```python
from build123d import *

# Parameters (mm, degrees)
F0_W     = 76.2
F0_H     = 254
F0_R     = 6.35
F1_DEPTH = 25.4
F2_R     = 38.09999


# Not quite as in the source:
# - a fillet or chamfer is up to 0.001 mm smaller than in the source, because OpenCascade refuses the exact size


with BuildPart() as f1:
    # F0 (on Front) → F1 (new body)
    with BuildSketch(Plane.XZ):
        with Locations((-38.1, 127)):
            Rectangle(F0_W, F0_H)
        with Locations((-38.1, 228.6)):
            Circle(F0_R, mode=Mode.SUBTRACT)
    extrude(amount=F1_DEPTH)

    # F2 (radius 38.1 in the source; OpenCascade refuses exactly that, so slightly less here)
    f2_edges = [f1.edges().sort_by_distance(p)[0] for p in [
        (-76.2, -12.7, 254),
        (0, -12.7, 254),
    ]]
    fillet(f2_edges, radius=F2_R)


solid = f1.part
```
Could you check a few things on this model? Use its own coordinates, in mm. Give positions to 0.01 mm unless a question says otherwise; leave off trailing zeros. Write each loop counter-clockwise with the first axis right and the second up, starting at its lowest first coordinate (ties: lowest second). Pieces come first, ordered by that corner, then holes. Notation, with made-up numbers: (-25, 73.25) -> (22, 73.25) arc R23 ccw to (22, 86.25) -> close; hole circle Ø7 at (9, 73.25). An arc over 180 degrees is marked (long way). Write each question's results on one line, items separated by ' | '.
1. I need wall thicknesses on L1, parallel to X at y = -18, z = 224.5; L2, parallel to Z at x = -58, y = -18; L3, parallel to Z at x = -36.5, y = -15.25. Which ranges of each line are inside material? Lowest first, please.
Check sheet entries:
L1: x = -75.22 to -42.95, -33.25 to -0.98 | L2: z = 0 to 248.39 | L3: z = 0 to 222.45, 234.75 to 253.97
2. I want a section at C-C, the plane x = -67. Write out the boundary of the cut face in (y, z).
Check sheet entries:
outline: (-25.4, 0) -> (0, 0) -> (0, 240.73) -> (-25.4, 240.73) -> close
3. I want a section at B-B, the plane z = 228.6. Write out the boundary of the cut face in (x, y), then the cut area to 3 significant figures.
Check sheet entries:
outline: (-74.02, -25.4) -> (-44.45, -25.4) -> (-44.45, 0) -> (-74.02, 0) -> close; (-31.75, -25.4) -> (-2.18, -25.4) -> (-2.18, 0) -> (-31.75, 0) -> close | area: 1,500 mm²
4. If we mould it in two halves opening along X, with no side actions, what happens to faces 1 (the cylindrical face through (-39.48, -12.52, 222.4)), 2 (the cylindrical face through (-11.46, -12.88, 243.14)), 3 (the flat face through (-39, 0, 129)), 4 (the flat face through (-76.2, -13, 106))? For each: released by +X, released by -X, zero draft, split by the parting line, or undercut.
Check sheet entries:
face 1: undercut | face 2: released by +X | face 3: zero draft | face 4: released by -X
5. I want a section at D-D, the plane x = -55. Write out the boundary of the cut face in (y, z), then the cut area to 3 significant figures.
Check sheet entries:
outline: (-25.4, 0) -> (0, 0) -> (0, 250.05) -> (-25.4, 250.05) -> close | area: 6,350 mm²
